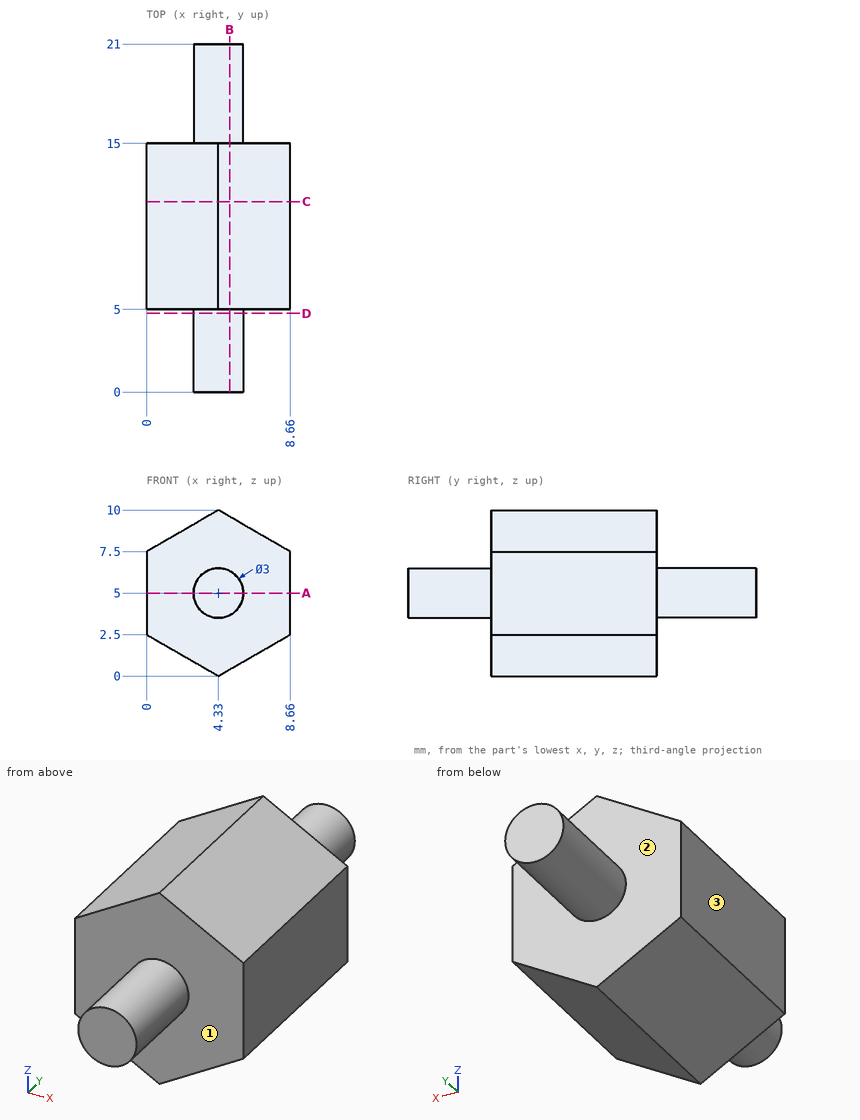
Design review of the part shown in the three views and the two pictorial views. Dimensions are in mm from the part's minimum x, y and z. A direction names the side the tool comes from. Coordinates: 2 decimals unless noted, no trailing zeros. Order: outer loops, then holes, each group sorted by start corner. A loop starts at its lowest first (then second) coordinate and runs counter-clockwise, first axis right, second up.
Item 1: Take a section at B-B, the plane x = 5. Write out the cut boundary in (y, z), then the cut area to 3 significant figures.
Item 2: Take a section at A-A, the plane z = 5. Write out the cut boundary in (x, y), then the cut area to 3 significant figures.
Item 3: Take a section at D-D, the plane y = 4.75. Write out the cut boundary in (x, z).
Item 4: For line 1 (Y direction, x = 6.25, z = 3); line 2 (X direction, y = 19, z = 5.5) (1 decimal); line 3 (Z direction, x = 3.25, y = 6.5), list the stretches that pass through material, from the lowest coordinate up.
Item 5: For the marked faces 1, 2 and 3, list the 3-axis set-ups (+Z, -Z, +X, -X, +Y, -Y) from which the entire face can be reached by the end or side of a thin tool; tool diameter is ignored.
Item 6: Take a section at C-C, the plane y = 11.5. Write out the cut boundary in (x, z).
Item 7: For pin 1 Ø4 at (x, y) = (2, 13) entering from -Z; pin 2 Ø2 at (x, y) = (3.5, 18.5) entering from +Z; pin 3 Ø1.5 at (x, z) = (1, 4) entering from -Y, all flat-tipped, find the tip position at first contact; note any pin that passes through.
The answers:
1. outline: (0, 3.66) - (5, 3.66) - (5, 0.39) - (15, 0.39) - (15, 3.66) - (21, 3.66) - (21, 6.34) - (15, 6.34) - (15, 9.61) - (5, 9.61) - (5, 6.34) - (0, 6.34) - close
1. area: 122 mm2
2. outline: (0, 5) - (2.83, 5) - (2.83, 0) - (5.83, 0) - (5.83, 5) - (8.66, 5) - (8.66, 15) - (5.83, 15) - (5.83, 21) - (2.83, 21) - (2.83, 15) - (0, 15) - close
2. area: 120 mm2
3. outline: circle Ø3 at (4.33, 5)
4. line 1: y = 5 to 15
4. line 2: x = 2.9 to 5.7
4. line 3: z = 0.62 to 9.38
5. face 1: -Y
5. face 2: +Y
5. face 3: +Z, -Z, -X, +Y, -Y
6. outline: (0, 2.5) - (4.33, 0) - (8.66, 2.5) - (8.66, 7.5) - (4.33, 10) - (0, 7.5) - close
7. pin 1: stops at z = 0.19
7. pin 2: stops at z = 6.5
7. pin 3: stops at y = 5
